from build123d import *

# Parameters (mm, degrees)
F0_R     = 5
F0_R_2   = 2.25
F1_DEPTH = 20
F2_R     = 2
F3_R     = 7
F3_R_2   = 2.25
F4_DEPTH = 2


with BuildPart() as f1:
    # F0 (on Top) → F1 (new body)
    with BuildSketch(Plane.XY):
        Circle(F0_R)
        Circle(F0_R_2, mode=Mode.SUBTRACT)
    extrude(amount=-F1_DEPTH)

    # F2
    f2_edges = [f1.edges().sort_by_distance(p)[0] for p in [
        (-5, 0, -20),
    ]]
    fillet(f2_edges, radius=F2_R)

    # F3 (on face) → F4 (join)
    with BuildSketch(Plane.XY):
        Circle(F3_R)
        Circle(F3_R_2, mode=Mode.SUBTRACT)
    extrude(amount=F4_DEPTH)


solid = f1.part
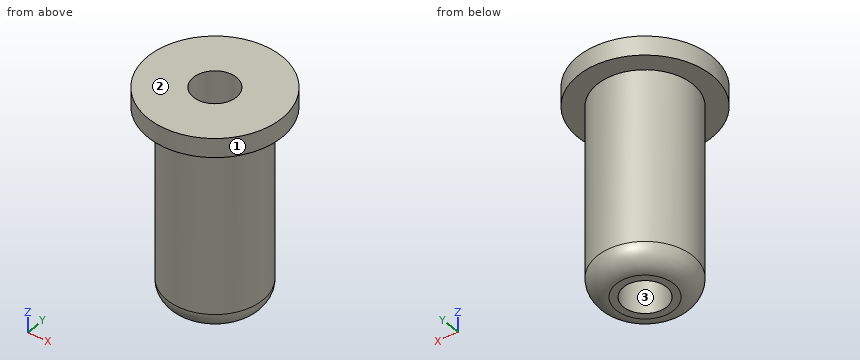
Can you work these out from the model? Positions are in its coordinate system, mm. Face numbers are marked on the shaded views. Round coordinates to 2 decimals unless told otherwise and drop trailing zeros. Write each loop counter-clockwise with the first axis right and the second up, starting at its lowest first coordinate (ties: lowest second). Pieces come first, ordered by that corner, then holes. Notation, with made-up numbers: M 44.5,57 L 93.5,57 A23 ccw 93.5,86 Z; hole C 27.25,17 d1. An arc over 180 degrees is marked long. Use CSV: the item, a comma, the result in double quotes.
(1) I need wall thicknesses on line 1 along Y through (x, z) = (0, -4); line 2 along Y through (x, z) = (0.75, -2.5); line 3 along Z through (x, y) = (5, 4.25). Which ranges of each line are inside material? Lowest first, please.
Check values:
line 1,"-5 to -2.25, 2.25 to 5"
line 2,"-4.94 to -2.12, 2.12 to 4.94"
line 3,"0 to 2"
(2) We'd pull the mould along X, two halves only. Please class the marked faces 1, 2 and 3: +X half, -X half, draft (parallel to the pull), parting line (faces both ways), or undercut.
Check values:
face 1,"parting line"
face 2,"draft"
face 3,"undercut"
(3) Imagine slicing it at A-A (x = 0). Write out the boundary of the cut face in (y, z).
Check values:
outline,"M -7,0 L -5,0 L -5,-18 A2 ccw -3,-20 L -2.25,-20 L -2.25,2 L -7,2 Z; M 2.25,-20 L 3,-20 A2 ccw 5,-18 L 5,0 L 7,0 L 7,2 L 2.25,2 Z"
(4) I'm going to push flat-ended pins straight in: pin 1 (1 mm diameter, centred on y = -5, z = -10.5, fed in from +X); pin 2 (2 mm diameter, centred on x = -3, z = -9.5, fed in from -Y); pin 3 (4 mm diameter, centred on x = -3.5, z = -18, fed in from +Y); pin 4 (3.5 mm diameter, centred on x = 0, y = 0, fed in from +Z). Where does each tip first touch, or does it pass through?
Check values:
pin 1,"x = 2.18"
pin 2,"y = -4.58"
pin 3,"y = 4.77"
pin 4,"through"
(5) Imagine slicing it at C-C (z = -9.5). Write out the boundary of the cut face in (x, y).
Check values:
outline,"C 0,0 d10; hole C 0,0 d4.5"
(6) Imagine slicing it at B-B (z = 0.25). Write out the boundary of the cut face in (x, y).
Check values:
outline,"C 0,0 d14; hole C 0,0 d4.5"
